Verification items for the finished model (mm, model axes). A direction names the side the tool comes from. Give positions to 0.01 mm unless a question says otherwise; leave off trailing zeros. Order: outer loops, then holes, each group sorted by start corner. A loop starts at its lowest first (then second) coordinate and runs counter-clockwise, first axis right, second up. Notation, with made-up numbers: (12, -6.5) -> (51, -6.5) arc R16 ccw to (51, 10.5) -> close; hole circle Ø3 at (30, 6). An arc over 180 degrees is marked (long way). Write each question's results on one line, items separated by ' | '. Start each with the question number.
1. Material ranges on L1, parallel to Y at x = -174, z = 14.5, recorded low to high. Write a range as from..to.
2. Mould release check, pull along X, two halves, no side actions. Record for faces 5 (the face through (37.878, -157, 9)), 6 (the face through (-3, 135, 0)), 7 (the face through (-1, -148.142, 9)), 8 (the face through (126.778, -157, 9)): +X half, -X half, draft (parallel to the pull), parting line (faces both ways), or undercut.
3. Set-up check for faces 1 (the face through (-38.322, -157, 9)), 2 (the face through (37.878, 420, 9)), 3 (the face through (-127.222, -157, 9)), 4 (the face through (164, 410.658, 9)): record each of +Z, -Z, +X, -X, +Y, -Y from which the full face is reachable in a straight line by a thin tool's end or side.
4. Depth check by flat-ended pin: pin 1 Ø4 at (x, z) = (-149, 10) entering from -Y; pin 2 Ø5.5 at (y, z) = (-154, 7.5) entering from +X; pin 3 Ø9.5 at (y, z) = (416.5, 12) entering from -X. Enter the tip coordinate at first touch or a pass-through.
5. Cross-section at A-A, the plane z = 3.5. Enter the section's corners in (x, y).
6. Cross-section at B-B, the plane x = 13. Enter the section's corners in (y, z).
from build123d import *

# Parameters (mm, degrees)
F0_W     = 406.4
F0_H     = 558.8
F1_DEPTH = 18.542
F2_W     = 88.9
F2_H     = 18.542
F3_DEPTH = 18.542
F4_W     = 88.9
F4_H     = 18.542
F5_DEPTH = 18.542


with BuildPart() as f1:
    # F0 (on Top) → F1 (new body)
    with BuildSketch(Plane.XY):
        with Locations((-0.222251, 131.257872)):
            Rectangle(F0_W, F0_H)
    extrude(amount=F1_DEPTH)

    # F2 (on face) → F3 (join)
    with BuildSketch(Plane.XZ.offset(148.142128)):
        with Locations((-82.772251, 9.271)):
            Rectangle(F2_W, F2_H)
        with Locations((82.327749, 9.271)):
            Rectangle(F2_W, F2_H)
    extrude(amount=F3_DEPTH)

    # F4 (on face) → F5 (join)
    with BuildSketch(Plane(origin=(0, 410.657872, 0), x_dir=(-1, 0, 0), z_dir=(0, 1, 0))):
        with Locations((-82.327749, 9.271)):
            Rectangle(F4_W, F4_H)
        with Locations((82.772251, 9.271)):
            Rectangle(F4_W, F4_H)
    extrude(amount=F5_DEPTH)


solid = f1.part
Results below:
1) L1: y = -148.14..410.66
2) face 5: undercut | face 6: draft | face 7: undercut | face 8: +X half
3) face 1: +Z, -Z, -Y | face 2: +Z, -Z, +Y | face 3: +Z, -Z, -X, -Y | face 4: +Z, -Z, +X, +Y
4) pin 1: stops at y = -148.14 | pin 2: stops at x = 126.78 | pin 3: stops at x = -127.22
5) outline: (-203.42, -148.14) -> (-127.22, -148.14) -> (-127.22, -166.68) -> (-38.32, -166.68) -> (-38.32, -148.14) -> (37.88, -148.14) -> (37.88, -166.68) -> (126.78, -166.68) -> (126.78, -148.14) -> (202.98, -148.14) -> (202.98, 410.66) -> (126.78, 410.66) -> (126.78, 429.2) -> (37.88, 429.2) -> (37.88, 410.66) -> (-38.32, 410.66) -> (-38.32, 429.2) -> (-127.22, 429.2) -> (-127.22, 410.66) -> (-203.42, 410.66) -> close
6) outline: (-148.14, 0) -> (410.66, 0) -> (410.66, 18.54) -> (-148.14, 18.54) -> close
